Here's how the part is built. I have some questions about the finished solid (model axes, mm). A direction names the side the tool comes from. Round coordinates to 2 decimals unless told otherwise and drop trailing zeros. Write each loop counter-clockwise with the first axis right and the second up, starting at its lowest first coordinate (ties: lowest second). Pieces come first, ordered by that corner, then holes. Notation, with made-up numbers: (27, -5) - (54, -5) arc R17 ccw to (54, 21) - close; hole circle Ø3 at (11.5, 63). An arc over 180 degrees is marked (long way). Use one line per item in the form item = value. Start each with the question number.
1. I want a section at B-B, the plane z = 29.5. List the corners of the cut face in (x, y) for me, plus the area to 3 significant figures.
2. We'd pull the mould along Y, two halves only. Please class faces 5 (the flat face through (47.89, 7.76, -0.78)), 6 (the cylindrical face through (61.6, -1.63, -17.64)), 7 (the conical face through (63.9, -3.6, -20.4)): +Y half, -Y half, draft (parallel to the pull), parting line (faces both ways), or undercut.
3. If I drill on line 1 along Z through (x, y) = (52.5, 5); line 2 along Z through (x, y) = (61.25, 3.75); line 3 along Z through (x, y) = (51.75, 2.75), over which ranges is the centre line in solid material (lowest first)?
4. Will these pins go through, and if not, where does the flat tip stop? pin 1 (10 mm diameter, centred on x = 50.5, z = 14.5, fed in from -Y); pin 2 (6 mm diameter, centred on x = 47, y = 5, fed in from +Z); pin 3 (6 mm diameter, centred on y = 7, z = -8, fed in from -X); pin 4 (6 mm diameter, centred on y = 9, z = 24, fed in from -X).
5. Which directions (+Z, -Z, +X, -X, +Y, -Y) give clear straight access to the entire face, cutting with the end or side of a thin tool? Please do faces 1 (the cylindrical face through (52.108, -1.521, -24.732)), 2 (the flat face through (49.512, -2.059, -2.505)), 3 (the flat face through (58.24, 6.22, -2.51)), 4 (the flat face through (58, -2, 52.5)).
```python
from build123d import *
from OCP.BRepFilletAPI import BRepFilletAPI_MakeChamfer

# Parameters (mm, degrees)
BOSS_EXTRUDE1_DEPTH      = 3
SKETCH4_R                = 6
BOSS_EXTRUDE2_DEPTH      = 40
BOSS_EXTRUDE3_DEPTH      = 4.7
BOSS_EXTRUDE3_DEPTH_BACK = 1.5
CHAMFER1_START           = -13.500000159
CHAMFER1_DEPTH           = 12.000000159
CHAMFER1_2_ANGLE         = 180
CUT_EXTRUDE1_DEPTH       = 3.4
SKETCH9_R                = 1.4
CUT_EXTRUDE2_DEPTH       = 27.5
SKETCH10_R               = 3.5
CUT_EXTRUDE3_DEPTH       = 23
CHAMFER2_SIZE            = 3
CHAMFER2_SIZE_2          = 2.517298894
CHAMFER3_SIZE            = 1
CHAMFER3_SIZE2           = 1.169832114
CHAMFER3_SIZE2_2         = 0.887609284
CHAMFER4_SIZE            = 1.732050808
CHAMFER4_SIZE_2          = 1
CHAMFER5_SIZE            = 0.3
CHAMFER5_SIZE2           = 0.289831366


with BuildPart() as part:
    # Sketch3 → Boss-Extrude1 (new body)
    with BuildSketch(Plane.XY):
        with BuildLine():
            ThreePointArc((-21.06925633, 1.560185503), (-21.702383426, -4.120337722), (-16.861546239, -7.159332517))
            Line((-16.861546239, -7.159332517), (-16.235942246, -7.122800897))
            ThreePointArc((-16.235942246, -7.122800897), (-14.247317716, -6.480760333), (-12.653836147, -5.128850538))
            ThreePointArc((-12.653836147, -5.128850538), (21.262556938, 11.81913919), (56.062735888, -3.230898045))
            ThreePointArc((56.062735888, -3.230898045), (59.548283557, -3.823314658), (60.140700171, -0.337766989))
            ThreePointArc((60.140700171, -0.337766989), (19.96998669, 19.192613792), (-21.06925633, 1.560185503))
        make_face()
        Polygon((-14.842971244, -1.436629161), (-14.495267888, -1.784332517), (-14.848821278, -2.137885908), (-14.637840313, -2.550832882), (-15.083092963, -2.778319315), (-15.00954079, -3.236171091), (-15.503211236, -3.315477399), (-15.574237606, -3.773727796), (-16.068337858, -3.697144889), (-16.277038544, -4.111248976), (-16.723538831, -3.886221213), (-17.049626765, -4.215925369), (-17.405124343, -3.864326917), (-17.816901648, -4.077581746), (-18.046839834, -3.633590269), (-18.504279068, -3.70966601), (-18.586306367, -3.21644038), (-19.04494145, -3.147941973), (-18.971084274, -2.65342694), (-19.386332882, -2.447012878), (-19.163770631, -1.999278532), (-19.495267888, -1.67501361), (-19.145635065, -1.317582653), (-19.361157273, -0.906987537), (-18.918440472, -0.674604591), (-18.997037466, -0.217591808), (-18.504271649, -0.132846012), (-18.438303288, 0.326159812), (-17.94338851, 0.255030612), (-17.73926735, 0.671411115), (-17.290312559, 0.451321143), (-16.967880508, 0.784601421), (-16.60852704, 0.436944858), (-16.199126599, 0.654727893), (-15.964305958, 0.213299227), (-15.507733522, 0.294415085), (-15.420271807, -0.197875935), (-14.960909199, -0.261312244), (-15.029308259, -0.756611718), (-14.611808522, -0.958433771), align=None, mode=Mode.SUBTRACT)
    extrude(amount=BOSS_EXTRUDE1_DEPTH)


with BuildPart() as body_2:
    # Sketch4 → Boss-Extrude2 (new, symmetric)
    with BuildSketch(Plane.XY.offset(12.5)):
        with Locations((58.101718029, -1.784332517)):
            Circle(SKETCH4_R)
    extrude(amount=BOSS_EXTRUDE2_DEPTH, both=True)

    # Sketch8 → Boss-Extrude3 (add, two sides: drawn at the far end of the back side and taken through both)
    with BuildSketch(Plane.XY.offset(-BOSS_EXTRUDE3_DEPTH_BACK)):
        with BuildLine():
            Line((62.151425867, 2.642841122), (51.244940369, 12.619427404))
            Line((51.244940369, 12.619427404), (44.360090975, 2.654069132))
            Line((44.360090975, 2.654069132), (54.052010192, -6.211506156))
            ThreePointArc((54.052010192, -6.211506156), (62.528891669, -5.834040354), (62.151425867, 2.642841122))
        make_face()
    extrude(amount=BOSS_EXTRUDE3_DEPTH + BOSS_EXTRUDE3_DEPTH_BACK)

    # Chamfer1: read off the stored shape, not the designer's step
    # Chamfer1 outline → Chamfer1 (add)
    with BuildSketch(Plane.XY.offset(CHAMFER1_START)):
        with BuildLine():
            Line((51.244940369, 12.619427404), (44.360090975, 2.654069132))
            Line((44.360090975, 2.654069132), (54.052010192, -6.211506156))
            ThreePointArc((54.052010192, -6.211506156), (53.67454439, 2.265375321), (62.151425867, 2.642841122))
            Line((62.151425867, 2.642841122), (51.244940369, 12.619427404))
        make_face()
    extrude(amount=CHAMFER1_DEPTH)

    # Chamfer1 2 outline → Chamfer1 2 (revolve, cut)
    with BuildSketch(Plane(origin=(58.101718029, -1.784332517, 0), x_dir=(0.6749513062060508, 0.7378622732263427, 0), z_dir=(0.7378622732263427, -0.6749513062060508, 0))):
        Polygon((15.952545244, -1.63901845), (5.999993338, -13.500007939), (15.952545243, -13.500000159), align=None)
    revolve(axis=Axis((58.101718029, -1.784332517, 0), (0, 0, 1)), revolution_arc=CHAMFER1_2_ANGLE, mode=Mode.SUBTRACT)

    # Sketch6 → Cut-Extrude1 (cut)
    with BuildSketch(Plane.XY):
        with BuildLine():
            Line((-16.85267585, -7.459325585), (-16.209835721, -7.421787475))
            ThreePointArc((-16.209835721, -7.421787475), (-14.1052834, -6.74504216), (-12.418987212, -5.315521311))
            ThreePointArc((-12.418987212, -5.315521311), (21.262849062, 11.519032134), (55.827922983, -3.418301943))
            ThreePointArc((55.827922983, -3.418301943), (59.733301775, -4.059840039), (60.378935523, -0.155136246))
            ThreePointArc((60.378935523, -0.155136246), (19.977496019, 19.492520208), (-21.298028536, 1.754487883))
            ThreePointArc((-21.298028536, 1.754487883), (-21.97276199, -4.250320867), (-16.85267585, -7.459325585))
        make_face()
    extrude(amount=CUT_EXTRUDE1_DEPTH, mode=Mode.SUBTRACT)

    # Sketch9 → Cut-Extrude2 (cut)
    with BuildSketch(Plane(origin=(0, 0, -27.5), x_dir=(-1, 0, 0), z_dir=(0, 0, -1))):
        with Locations((-58.101718029, -1.784332517)):
            Circle(SKETCH9_R)
    extrude(amount=-CUT_EXTRUDE2_DEPTH, mode=Mode.SUBTRACT)

    # Sketch10 → Cut-Extrude3 (cut)
    with BuildSketch(Plane(origin=(0, 0, -27.5), x_dir=(-1, 0, 0), z_dir=(0, 0, -1))):
        with Locations((-58.101718029, -1.784332517)):
            Circle(SKETCH10_R)
    extrude(amount=-CUT_EXTRUDE3_DEPTH, mode=Mode.SUBTRACT)

    # Chamfer2
    # the kernel refuses this chamfer: 3, 2.517298894 mm, written as the material it adds along each edge
    with BuildSketch(Plane(origin=(58.101718029, -1.784332517, -4.5), x_dir=(-1, 0, 0), z_dir=(0, -1, 0))) as chamfer2_piece_1_section:
        Polygon((3.5, CHAMFER2_SIZE), (3.5 - CHAMFER2_SIZE_2, 0), (3.5, 0), align=None)
    chamfer2_piece_1 = revolve(axis=Axis((58.101718029, -1.784332517, -4.5), (0, 0, -1)), mode=Mode.PRIVATE)
    chamfer2_piece_1 = chamfer2_piece_1 - Plane(origin=(58.101718029, -1.784332517, -4.5), x_dir=(-1, 0, 0), z_dir=(0, 0, -1)) * Cylinder(1.4, 14, mode=Mode.PRIVATE)
    add(chamfer2_piece_1)

    # Sketch11 → Revolve1 (revolve)
    with BuildSketch(Plane(origin=(58.101718029, 0, 0), x_dir=(0, 0, -1), z_dir=(1, 0, 0)), mode=Mode.PRIVATE) as revolve1_sk:
        Polygon((27.5, -7.784332517), (27.5, -8.784332517), (26, -7.784332517), align=None)
        Polygon((23.5, -7.784332517), (22, -8.784332517), (22, -7.784332517), align=None)
    revolve1 = revolve(revolve1_sk.sketch.rotate(Axis((58.101718029, -1.784332517, 52.5), (0, 0, -1)), 270), axis=Axis((58.101718029, -1.784332517, 52.5), (0, 0, -1)))

    # Mirror1: Revolve1 across plane
    add(revolve1.mirror(Plane.XY.offset(12.5)))

    # Chamfer3: one chamfer whose edges measure the first distance from different faces: ONE call of the kernel's chamfer builder (chamfer() names one face for all edges)
    chamfer3_edges_1 = [body_2.edges().sort_by_distance(p)[0] for p in [
        (44.360090975, 2.654069132, 1.6),
    ]]
    chamfer3_side_1 = [body_2.faces().sort_by_distance(p)[0] for p in [
        (49.206050583, -1.778718512, 1.6),
    ]]
    chamfer3_edges_2 = [body_2.edges().sort_by_distance(p)[0] for p in [
        (51.244940369, 12.619427404, 1.6),
    ]]
    chamfer3_side_2 = [body_2.faces().sort_by_distance(p)[0] for p in [
        (47.802515672, 7.636748268, 4.563930343),
    ]]
    chamfer3 = BRepFilletAPI_MakeChamfer(body_2.part.solid().wrapped)
    for e in chamfer3_edges_1:
        chamfer3.Add(CHAMFER3_SIZE, CHAMFER3_SIZE2, e.wrapped, chamfer3_side_1[0].wrapped)  # the first distance lies on this face
    for e in chamfer3_edges_2:
        chamfer3.Add(CHAMFER3_SIZE, CHAMFER3_SIZE2_2, e.wrapped, chamfer3_side_2[0].wrapped)  # the first distance lies on this face
    add(Compound.cast(chamfer3.Shape()), mode=Mode.REPLACE)

    # Chamfer4
    # the kernel refuses this chamfer: 1.732050808, 1 mm, written as the material it adds along each edge
    with BuildSketch(Plane(origin=(58.101718029, -1.784332517, -22), x_dir=(1, 0, 0), z_dir=(0, 1, 0))) as chamfer4_piece_1:
        Polygon((6, -CHAMFER4_SIZE), (6 + CHAMFER4_SIZE_2, 0), (6, 0), align=None)
    revolve(axis=Axis((58.101718029, -1.784332517, -22), (0, 0, -1)))
    with BuildSketch(Plane(origin=(58.101718029, -1.784332517, 47), x_dir=(1, 0, 0), z_dir=(0, 1, 0))) as chamfer4_piece_2:
        Polygon((6, CHAMFER4_SIZE), (6 + CHAMFER4_SIZE_2, 0), (6, 0), align=None)
    revolve(axis=Axis((58.101718029, -1.784332517, 47), (0, 0, -1)))

    # Chamfer5: one chamfer whose edges measure the first distance from different faces: ONE call of the kernel's chamfer builder (chamfer() names one face for all edges)
    chamfer5_edges_1 = [body_2.edges().sort_by_distance(p)[0] for p in [
        (51.101718029, -1.784332517, -27.5),
    ]]
    chamfer5_side_1 = [body_2.faces().sort_by_distance(p)[0] for p in [
        (61.799707928, -1.784332517, -27.5),
    ]]
    chamfer5_edges_2 = [body_2.edges().sort_by_distance(p)[0] for p in [
        (51.101718029, -1.784332517, 52.5),
    ]]
    chamfer5_side_2 = [body_2.faces().sort_by_distance(p)[0] for p in [
        (51.601718029, -1.784332517, 51.75),
    ]]
    chamfer5 = BRepFilletAPI_MakeChamfer(body_2.part.solid().wrapped)
    for e in chamfer5_edges_1:
        chamfer5.Add(CHAMFER5_SIZE, CHAMFER5_SIZE2, e.wrapped, chamfer5_side_1[0].wrapped)  # the first distance lies on this face
    for e in chamfer5_edges_2:
        chamfer5.Add(CHAMFER5_SIZE, CHAMFER5_SIZE2, e.wrapped, chamfer5_side_2[0].wrapped)  # the first distance lies on this face
    add(Compound.cast(chamfer5.Shape()), mode=Mode.REPLACE)


solid = body_2.part
```
Model answer:
q1.outline = circle Ø12 at (58.1, -1.78)
q1.area = 113 mm2
q2.face_5 = +Y half
q2.face_6 = undercut
q2.face_7 = parting line
q3.line_1 = -10.17 to 0, 3.4 to 4.7
q3.line_2 = -27.5 to -26.55, -22.95 to -20.9, 45.9 to 47.95, 51.55 to 52.5
q3.line_3 = -11.35 to 0, 3.4 to 4.7
q4.pin_1 = -7.19
q4.pin_2 = 4.7
q4.pin_3 = 47.57
q4.pin_4 = through
q5.face_1 = none
q5.face_2 = -X, -Y
q5.face_3 = +X, +Y
q5.face_4 = +Z, +X, -X, +Y, -Y
